Build history of the part. All positions in model axes, mm. Coordinates: 2 decimals unless noted, no trailing zeros. Loops run counter-clockwise (first coordinate to the right, second up) from the corner with the lowest first, then second, coordinate; pieces in that order, holes last.
Item 1: Flat gauge pins, fed straight in: pin 1 (0.9 mm diameter, centred on x = 21.5, z = -1.5, fed in from -Y); pin 2 (1.2 mm diameter, centred on x = 135.5, y = -128.5, fed in from +Z); pin 3 (1.5 mm diameter, centred on x = 128.5, z = -1.5, fed in from -Y). Where does each tip first touch, or does it go through?
Item 2: Cut at C-C (y = -30). List the corners of the cut face in (x, z), and give its area (3 significant figures).
Item 3: Drill centre lines: line 1 along Z through (x, y) = (45, -32); line 2 along X through (y, z) = (-49.5, -1.7); line 3 along Y through (x, z) = (88, -1.5). Where is each one in solid material? Low to high.
Item 4: Cut at A-A (z = 0.9). Count the separate pieces of the cut face and the enclosed holes in it, and give its area (3 significant figures).
Item 5: Cut at B-B (x = 61). List the corners of the cut face in (y, z).
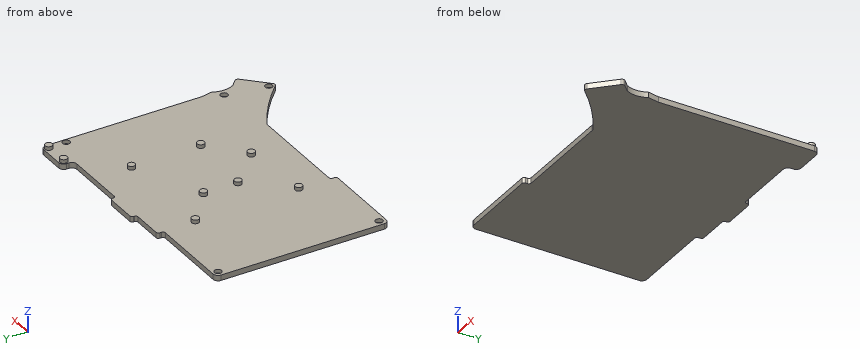
from build123d import *

# Parameters (mm, degrees)
PAD_DEPTH       = 3
SKETCH013_R     = 1.970107
SKETCH013_R_2   = 2.014006
SKETCH013_R_3   = 1.966045
SKETCH013_R_4   = 2.046443
SKETCH013_R_5   = 1.971077
SKETCH013_R_6   = 2.0005
SKETCH013_R_7   = 2.019658
SKETCH013_R_8   = 1.997918
PAD014_DEPTH    = 2
SKETCH016_R     = 2
POCKET001_DEPTH = 2


with BuildPart() as part:
    # Sketch → Pad (new body)
    with BuildSketch(Plane.XY):
        with BuildLine():
            ThreePointArc((2.691092, -17.424324), (0.807563, -18.209051), (0.022899, -20.092606))
            Line((0.022899, -20.092606), (0.022899, -110.261101))
            ThreePointArc((0.022899, -110.261101), (0.80276, -112.148767), (2.690309, -112.928909))
            Line((2.690309, -112.928909), (46.758133, -112.928909))
            ThreePointArc((46.758133, -112.928909), (47.657861, -112.558702), (48.026189, -111.658203))
            Line((48.026189, -111.658203), (48.026189, -110.643822))
            ThreePointArc((49.299188, -109.370278), (48.401516, -109.74599), (48.026189, -110.643822))
            Line((49.299188, -109.370278), (105.051811, -109.370278))
            ThreePointArc((107.084557, -110.008187), (106.115549, -109.538299), (105.051811, -109.370278))
            ThreePointArc((134.00774, -130.962361), (121.270775, -119.55423), (107.084557, -110.008187))
            ThreePointArc((134.00774, -130.962361), (135.023899, -131.385154), (136.040024, -130.96228))
            Line((136.040024, -130.96228), (147.850815, -119.15155))
            ThreePointArc((147.850815, -119.15155), (148.27253, -118.135527), (147.850845, -117.119492))
            Line((147.850845, -117.119492), (144.422364, -113.692703))
            ThreePointArc((144.421555, -102.010086), (142.938996, -107.851497), (144.422364, -113.692703))
            Line((144.421555, -102.010086), (143.278885, -95.909729))
            Line((143.278885, -95.909729), (143.278885, -9.814656))
            ThreePointArc((143.278885, -9.814656), (142.501515, -7.922142), (140.611955, -7.137621))
            Line((140.611955, -7.137621), (126.896004, -7.137621))
            ThreePointArc((126.896004, -7.137621), (125.009764, -7.926259), (124.228843, -9.815708))
            Line((124.228843, -9.815708), (124.228843, -11.201195))
            ThreePointArc((121.560973, -13.869035), (123.447403, -13.087617), (124.228843, -11.201195))
            Line((121.560973, -13.869035), (87.398842, -13.869035))
            ThreePointArc((86.128205, -12.598599), (86.501641, -13.495741), (87.398842, -13.869035))
            Line((86.128205, -12.217462), (86.128205, -12.598599))
            ThreePointArc((86.128205, -12.217462), (85.757691, -11.31862), (84.859047, -10.947623))
            Line((84.859047, -10.947623), (68.094903, -10.947623))
            ThreePointArc((68.094903, -10.947623), (67.198822, -11.321427), (66.825078, -12.217532))
            Line((66.825078, -12.598418), (66.825078, -12.217532))
            ThreePointArc((65.554496, -13.868415), (66.453928, -13.497679), (66.825078, -12.598418))
            Line((65.554496, -13.868415), (49.045334, -13.868415))
            ThreePointArc((49.045334, -13.868415), (48.149198, -14.2429), (47.774544, -15.138965))
            Line((47.774544, -15.138965), (47.774544, -16.154249))
            ThreePointArc((46.504146, -17.424324), (47.403928, -17.053937), (47.774544, -16.154249))
            Line((46.504146, -17.424324), (2.691092, -17.424324))
        make_face()
    extrude(amount=-PAD_DEPTH)

    # Sketch013 → Pad014 (join)
    with BuildSketch(Plane.XY):
        with Locations((105.029465, -34.063732)):
            Circle(SKETCH013_R)
        with Locations((85.981422, -88.730209)):
            Circle(SKETCH013_R_2)
        with Locations((47.866016, -91.887985)):
            Circle(SKETCH013_R_3)
        with Locations((47.861008, -34.833092)):
            Circle(SKETCH013_R_4)
        with Locations((66.937889, -69.828568)):
            Circle(SKETCH013_R_5)
        with Locations((66.903061, -50.778069)):
            Circle(SKETCH013_R_6)
        with Locations((126.901398, -9.81155)):
            Circle(SKETCH013_R_7)
        with Locations((140.602615, -9.81155)):
            Circle(SKETCH013_R_8)
        with Locations((105.012505, -72.27108)):
            Circle(SKETCH013_R_2)
    extrude(amount=PAD014_DEPTH)

    # Sketch016 → Pocket001 (cut)
    with BuildSketch(Plane.XY):
        with Locations((135.15451, -128.047943)):
            Circle(SKETCH016_R)
        with Locations((139.153137, -105.817932)):
            Circle(SKETCH016_R)
        with Locations((140.994141, -19.711058)):
            Circle(SKETCH016_R)
        with Locations((3.483953, -109.468971)):
            Circle(SKETCH016_R)
        with Locations((3.485333, -20.56954)):
            Circle(SKETCH016_R)
    extrude(amount=-POCKET001_DEPTH, mode=Mode.SUBTRACT)


solid = part.part
Filled sheet:
1. pin 1: stops at y = -112.93
1. pin 2: stops at z = -2
1. pin 3: stops at y = -126.32
2. outline: (0.02, -3) - (143.28, -3) - (143.28, 0) - (0.02, 0) - close
2. area: 430 mm2
3. line 1: z = -3 to 0
3. line 2: x = 0.02 to 143.28
3. line 3: y = -109.37 to -13.87
4. separate pieces: 9
4. enclosed holes: 0
4. area: 113 mm2
5. outline: (-109.37, -3) - (-13.87, -3) - (-13.87, 0) - (-109.37, 0) - close
